Check sheet for the modelled part. Datum: model origin and axes. Units: mm. A direction names the side the tool comes from. Coordinates: 2 decimals unless noted, no trailing zeros. Write each loop counter-clockwise with the first axis right and the second up, starting at its lowest first coordinate (ties: lowest second). Pieces come first, ordered by that corner, then holes. Notation, with made-up numbers: (67.25, 68.5) -> (102.25, 68.5) arc R35 cw to (102.25, 103.5) -> close; hole circle Ø11 at (29.5, -24.75). An arc over 180 degrees is marked (long way). One line per item, written item: value. Start each with the question number.
1) Gauge pin test, flat ends, axial feed: P1, Ø1.5, axis at y = -4.5, z = 0, coming from the +X side; P2, Ø1.1, axis at x = 0.5, z = 0, coming from the -Y side. Record the tip position at first contact, or that the pin passes through.
2) Sectioned sample at C-C on y = -11.75. Enter the section's corners in (x, z), plus the area to 3 significant figures.
3) Sectioned sample at D-D on z = -1.27. Enter the section's corners in (x, y).
4) Sectioned sample at B-B on x = 0. Enter the section's corners in (y, z) (3 decimals).
5) Set-up check for faces 1 (the flat face through (0, 0.5, 1.595)), 2 (the cylindrical face through (1.5, 2.42, 0.07)): record each of +Z, -Z, +X, -X, +Y, -Y from which the full face is reachable in a straight line by a thin tool's end or side.
6) Scan lines: line 1 along Y through (x, z) = (-0.4, -1.55); line 2 along Y through (x, z) = (0.2, -0.05); line 3 along X through (y, z) = (-15, 1.4). Record each from-to range of solid material in increasing order. Write a range as [from, to].
7) Sectioned sample at A-A on z = 0. Enter the section's corners in (x, y) (3 decimals).
Autodesk Inventor part; units mm, degrees
ref_plane "YZ Plane" through (0, 0, 0) normal (1, 0, 0) x (0, 1, 0)
ref_plane "XZ Plane" through (0, 0, 0) normal (0, 1, 0) x (-1, 0, 0)
ref_plane "XY Plane" through (0, 0, 0) normal (0, 0, 1) x (1, 0, 0)
sketch "Sketch1" plane through (0, 0, 0) normal (0, 0, 1) x (1, 0, 0)
  line L0 (0, 0) -> (1.925, 0)
  line L1 (1.925, 0) -> (1.925, 1)
  line L2 (1.925, 1) -> (1.5, 1)
  line L3 (1.5, 1) -> (1.5, 3.8)
  line L4 (0, 5.3) -> (0, 5.3)
  line L5 (0, 0) -> (-1.925, 0)
  line L6 (-1.925, 0) -> (-1.925, 1)
  line L7 (-1.925, 1) -> (-1.5, 1)
  line L8 (-1.5, 1) -> (-1.5, 3.8)
  line L9 (0, 5.3) -> (0, 5.3)
  arc A0 (0, 5.3) -> (-1.5, 3.8) centre (0, 3.8) ccw
  arc A1 (1.5, 3.8) -> (0, 5.3) centre (0, 3.8) ccw
  line L10 (0, 5.3) -> (0, 0)
  point P0 (1.5, 5.3)
  dimension "d0" = 1.925
  dimension "d1" = 1
  dimension "d2" = 0.425
  dimension "d3" = 4.3
  dimension "d4" = 1.5
  dimension "d5" = 1.925
  dimension "d6" = 0.425
  dimension "d7" = 1.5
revolve "Revolution1" add sketch "Sketch1" angle 360 about axis through (0, 5.3, 0) along (0, -1, 0) contours L5 L6 L7 L8 A0 L10
sketch "Sketch2" plane through (0, 0, 0) normal (0, -1, 0) x (1, 0, 0)
  circle A0 centre (0, 1.27) radius 0.25
  circle A1 centre (0, -1.27) radius 0.25
  line L0 (0, -1.02) -> (0, 1.02)
  point P0 (0, 0)
  point P1 (0, 0)
  dimension "d10" = 0.5
  dimension "d9" = 2.04
extrude "Extrusion1" add sketch "Sketch2" along normal blind 18 contours A0
extrude "Extrusion2" add sketch "Sketch2" along normal blind 15 contours A1
sketch "Sketch3" plane through (0, 1, 0) normal (0, 1, 0) x (1, 0, 0)
  circle A0 centre (0, 0) radius 1.5
  circle A1 centre (0, -1.27) radius 0.25
  circle A2 centre (0, 0) radius 1.925
  circle A3 centre (0, 0) radius 1.5
  circle A4 centre (0, 0) radius 1.925
  arc A5 (-1.0778, -1.595) -> (1.0778, -1.595) centre (0, 0) ccw
  line L0 (1.0778, -1.595) -> (-1.0778, -1.595)
  line L1 (0, -1.52) -> (0, -1.595)
  point P0 (0, 0)
  dimension "d17" = 0.075
extrude "Extrusion3" cut sketch "Sketch3" against normal up to surface (1 mm away) contours L0 A2 picked at (0.5832, -1.6646)
properties part number "LED" material "Polycarbonate, Clear"
Answers:
1. P1: passes through
1. P2: stops at y = 0
2. outline: circle Ø0.5 at (0, -1.27); circle Ø0.5 at (0, 1.27)
2. area: 0.393 mm2
3. outline: (-1.45, 0) -> (-0.25, 0) -> (-0.25, -15) -> (0.25, -15) -> (0.25, 0) -> (1.45, 0) -> (1.45, 1) -> (0.8, 1) -> (0.8, 3.8) arc R0.8 ccw to (-0.8, 3.8) -> (-0.8, 1) -> (-1.45, 1) -> close
4. outline: (-18, 1.02) -> (0, 1.02) -> (0, -1.02) -> (-15, -1.02) -> (-15, -1.52) -> (0, -1.52) -> (0, -1.925) -> (1, -1.925) -> (1, -1.5) -> (3.8, -1.5) arc R1.5 ccw to (3.8, 1.5) -> (1, 1.5) -> (1, 1.595) -> (0, 1.595) -> (0, 1.52) -> (-18, 1.52) -> close
5. face 1: +Z, +X, -X, +Y, -Y
5. face 2: +Y
6. line 1: y = [0, 1]
6. line 2: y = [0, 5.29]
6. line 3: x = [-0.21, 0.21]
7. outline: (-1.925, 0) -> (1.925, 0) -> (1.925, 1) -> (1.5, 1) -> (1.5, 3.8) arc R1.5 ccw to (-1.5, 3.8) -> (-1.5, 1) -> (-1.925, 1) -> close
